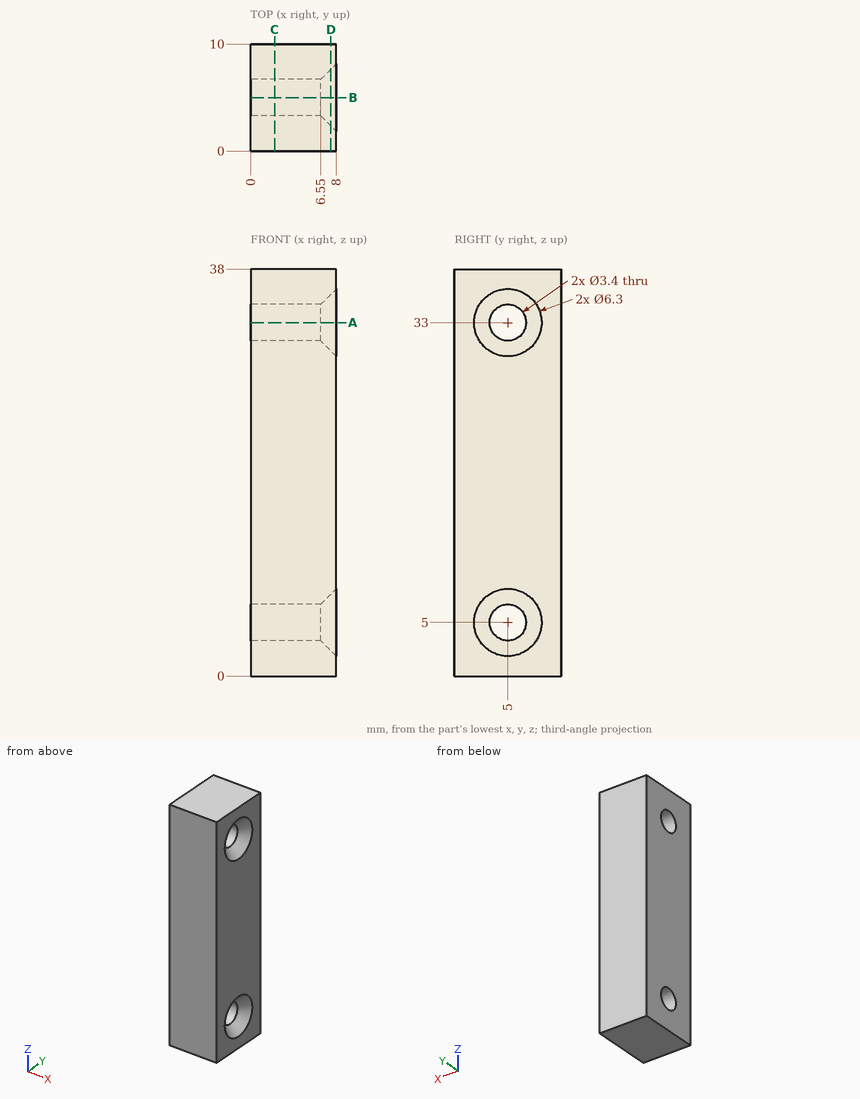
Source: three-view drawing plus pictorial views. Frame: mm from the lowest corner of the part. Coordinates: 2 decimals unless noted, no trailing zeros. Order: outer loops, then holes, each group sorted by start corner. A loop starts at its lowest first (then second) coordinate and runs counter-clockwise, first axis right, second up. Notation, with made-up numbers: M 85.25,88 L 99.25,88 A17 cw 99.25,112 Z; hole C 37.5,69.25 d4. An arc over 180 degrees is marked long. Answer in a Markdown table with one row per item.
(1) Section query D-D, the plane x = 7.5. Output: boundary loops of the cut face in (y, z).
Numbers:
| item | result |
|---|---|
| outline | M 0,0 L 10,0 L 10,38 L 0,38 Z; hole C 5,5 d5.3; hole C 5,33 d5.3 |
(2) Material intervals for line 1 (Z direction, x = 5.25, y = 5); line 2 (Y direction, x = 5.25, z = 33); line 3 (Z direction, x = 0.75, y = 4.5), sorted ascending. Write a range as [from, to].
Numbers:
| item | result |
|---|---|
| line 1 | z = [0, 3.3], [6.7, 31.3], [34.7, 38] |
| line 2 | y = [0, 3.3], [6.7, 10] |
| line 3 | z = [0, 3.38], [6.62, 31.38], [34.62, 38] |
(3) Section query B-B, the plane y = 5. Output: boundary loops of the cut face in (x, z).
Numbers:
| item | result |
|---|---|
| outline | M 0,0 L 8,0 L 8,1.85 L 6.55,3.3 L 0,3.3 Z; M 0,6.7 L 6.55,6.7 L 8,8.15 L 8,29.85 L 6.55,31.3 L 0,31.3 Z; M 0,34.7 L 6.55,34.7 L 8,36.15 L 8,38 L 0,38 Z |
(4) Contact query for a flat-ended pin moving along its axis: pin 1 Ø4 at (y, z) = (5, 33) entering from +X. Output: stop coordinate, or through.
Numbers:
| item | result |
|---|---|
| pin 1 | stops at x = 6.85 |
(5) Section query C-C, the plane x = 2.25. Output: boundary loops of the cut face in (y, z).
Numbers:
| item | result |
|---|---|
| outline | M 0,0 L 10,0 L 10,38 L 0,38 Z; hole C 5,5 d3.4; hole C 5,33 d3.4 |
(6) Section query A-A, the plane z = 33. Output: boundary loops of the cut face in (x, y).
Numbers:
| item | result |
|---|---|
| outline | M 0,0 L 8,0 L 8,1.85 L 6.55,3.3 L 0,3.3 Z; M 0,6.7 L 6.55,6.7 L 8,8.15 L 8,10 L 0,10 Z |
